from build123d import *

# Parameters (mm, degrees)
F1_DEPTH = 10.0076
F2_W     = 50.8
F2_H     = 25.4
F3_DEPTH = 10.0086
F4_R     = 76.2
F5_DEPTH = 10.0086


with BuildPart() as f1:
    # F0 (on Front) → F1 (new body)
    with BuildSketch(Plane.XZ):
        Polygon((711.428056, 899.191029), (-507.771944, 899.191029), (-507.771944, -1056.608971), (711.174056, -1056.608971), (711.174056, -320.008971), (711.428056, -320.008971), align=None)
    extrude(amount=F1_DEPTH)

    # F2 (on face) → F3 (cut, through all)
    with BuildSketch(Plane.XZ.offset(10.0076)):
        with Locations((686.028056, 886.491029)):
            Rectangle(F2_W, F2_H)
        with Locations((-482.371944, 886.491029)):
            Rectangle(F2_W, F2_H)
        with Locations((686.028056, -307.308971)):
            Rectangle(F2_W, F2_H)
        with Locations((-482.371944, -307.308971)):
            Rectangle(F2_W, F2_H)
        with Locations((-12.471944, -307.308971)):
            Rectangle(F2_W, F2_H)
    extrude(amount=-F3_DEPTH, mode=Mode.SUBTRACT)

    # F4 (on face) → F5 (cut, through all)
    with BuildSketch(Plane.XZ.offset(10.0076)):
        with Locations((-101.371944, 594.391029)):
            Circle(F4_R)
    extrude(amount=-F5_DEPTH, mode=Mode.SUBTRACT)


solid = f1.part
Geometry: final body of the model. Coordinates: model frame, mm. Give positions to 0.01 mm unless a question says otherwise; leave off trailing zeros. Loops run counter-clockwise (first coordinate to the right, second up) from the corner with the lowest first, then second, coordinate; pieces in that order, holes last. Notation, with made-up numbers: (35, 69.5) -> (51, 69.5) arc R23 cw to (51, 108.5) -> close; hole circle Ø4 at (28, -31). An arc over 180 degrees is marked (long way). Put each result on its own line as item: value.
1. Pull-direction query (Z, two-part tool) for faces 1 (the flat face through (93, -10.008, -65)), 2 (the cylindrical face through (-28.69, -5.07, 617.28)); classes: released by +Z, released by -Z, zero draft, split by the parting line, or undercut.
Taken from the geometry:
face 1: zero draft
face 2: undercut
2. Pin query (flat end, axial travel): P1, Ø3, axis at y = -7, z = 884, coming from the -X side; P2, Ø5, axis at y = -7, z = -708.5, coming from the +X side; P3, Ø5, axis at y = -5, z = -302, coming from the +X side. Return the tip coordinate at first contact, or that it passes through.
Taken from the geometry:
P1: stops at x = -456.97
P2: stops at x = 711.17
P3: stops at x = 660.63
3. Ray query, line 1 along Z through (x, y) = (-5, -6); line 2 along X through (y, z) = (-3, 596); line 3 along X through (y, z) = (-5.5, 661.5). Return the intervals inside material, ascending. Write a range as [from, to].
Taken from the geometry:
line 1: z = [-1056.61, -320.01], [-294.61, 899.19]
line 2: x = [-507.77, -177.55], [-25.19, 711.43]
line 3: x = [-507.77, -137.47], [-65.28, 711.43]
4. Cut plane A-A (x = -149.5). Return the cut outline in (y, z).
Taken from the geometry:
outline: (-10.01, -1056.61) -> (0, -1056.61) -> (0, 535.31) -> (-10.01, 535.31) -> close; (-10.01, 653.47) -> (0, 653.47) -> (0, 899.19) -> (-10.01, 899.19) -> close
